Build history of the part. All positions in model axes, mm. Face numbers are marked on the shaded views. Round coordinates to 2 decimals unless told otherwise and drop trailing zeros. Loops run counter-clockwise (first coordinate to the right, second up) from the corner with the lowest first, then second, coordinate; pieces in that order, holes last. Notation, with made-up numbers: (-23.75, 35) - (18.25, 35) arc R12 ccw to (18.25, 53) - close; hole circle Ø6 at (-11.75, -11). An arc over 180 degrees is marked (long way). Use a Markdown table: item, result.
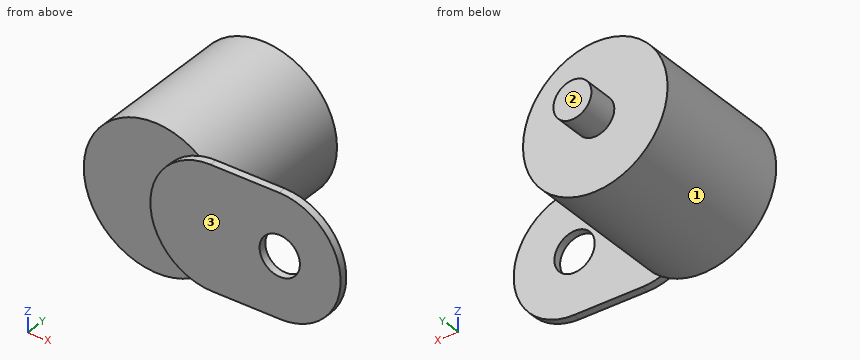
from build123d import *

# Parameters (mm, degrees)
SKETCH1_R           = 9.5
SKETCH1_R_2         = 2.5
BOSS_EXTRUDE1_DEPTH = 19
SKETCH2_R           = 2.5
BOSS_EXTRUDE2_DEPTH = 4
SKETCH3_R           = 2.65
BOSS_EXTRUDE3_DEPTH = 1


with BuildPart() as part:
    # Sketch1 → Boss-Extrude1 (new body)
    # profile 1 of 2: a face of its own
    with BuildSketch(Plane(origin=(0, 0, 0), x_dir=(1, 0, 0), z_dir=(0, 1, 0))):
        with Locations(Location((0, 0, 0), (0, 0, 270))):
            Circle(SKETCH1_R)
        Circle(SKETCH1_R_2, mode=Mode.SUBTRACT)
    # profile 2 of 2: a face of its own
    with BuildSketch(Plane(origin=(0, 0, 0), x_dir=(1, 0, 0), z_dir=(0, 1, 0))):
        Circle(SKETCH1_R_2)
    extrude(amount=BOSS_EXTRUDE1_DEPTH)

    # Sketch2 → Boss-Extrude2 (add)
    with BuildSketch(Plane(origin=(0, 19, 0), x_dir=(1, 0, 0), z_dir=(0, 1, 0))):
        with Locations(Location((0, 0, 0), (0, 0, 270))):
            Circle(SKETCH2_R)
    extrude(amount=BOSS_EXTRUDE2_DEPTH)

    # Sketch3 → Boss-Extrude3 (add)
    with BuildSketch(Plane.XZ):
        with BuildLine():
            Line((7.903037426, 7.99941237), (16.903037426, 8.108503279))
            ThreePointArc((16.903037426, 8.108503279), (24.99941237, 0.206053483), (17.096962574, -7.890321461))
            Line((17.096962574, -7.890321461), (8.096962574, -7.99941237))
            ThreePointArc((8.096962574, -7.99941237), (0.00058763, -0.096962574), (7.903037426, 7.99941237))
        make_face()
        with Locations(Location((17, 0.109090909, 0), (0, 0, 270))):
            Circle(SKETCH3_R, mode=Mode.SUBTRACT)
    extrude(amount=BOSS_EXTRUDE3_DEPTH)


solid = part.part
Q1. Probe line 1 (Y direction, x = -0.5, z = 4); line 2 (Y direction, x = 15, z = -5); line 3 (X direction, y = 15.75, z = -3). List the from-to ranges inside material, lowest first.
Results found:
| item | result |
|---|---|
| line 1 | y = 0 to 19 |
| line 2 | y = -1 to 0 |
| line 3 | x = -9.01 to 9.01 |
Q2. Cut at B-B, the plane x = -2. List the corners of the cut face in (y, z).
Results found:
| item | result |
|---|---|
| outline | (0, -9.29) - (19, -9.29) - (19, -1.5) - (23, -1.5) - (23, 1.5) - (19, 1.5) - (19, 9.29) - (0, 9.29) - close |
Q3. Cut at D-D, the plane y = 21. List the corners of the cut face in (x, z).
Results found:
| item | result |
|---|---|
| outline | circle Ø5 at (0, 0) |
Q4. Pull direction Y, two halves, no side cores. Call the marked faces 1, 2 and 3: pulls with the +Y half, pulls with the -Y half, needs draft (parallel to the pull), parting line crosses it, or undercut.
Results found:
| item | result |
|---|---|
| face 1 | needs draft |
| face 2 | pulls with the +Y half |
| face 3 | pulls with the -Y half |
Q5. Cut at A-A, the plane z = 0. List the corners of the cut face in (x, y), plus the area to 3 significant figures.
Results found:
| item | result |
|---|---|
| outline | (-9.5, 0) - (0, 0) - (0, -1) - (14.35, -1) - (14.35, 0) - (9.5, 0) - (9.5, 19) - (2.5, 19) - (2.5, 23) - (-2.5, 23) - (-2.5, 19) - (-9.5, 19) - close; (19.65, -1) - (25, -1) - (25, 0) - (19.65, 0) - close |
| area | 401 mm2 |
Q6. Drop flat-ended pins along their axis: pin 1 (5.5 mm diameter, centred on x = 0.5, z = 4, fed in from +Y); pin 2 (1.5 mm diameter, centred on x = 14, z = -5.5, fed in from +Y); pin 3 (5 mm diameter, centred on y = 6.5, z = -6, fed in from +X); pin 4 (2 mm diameter, centred on x = 1.5, z = -4.5, fed in from +Y). Give the stop position or say it passes through.
Results found:
| item | result |
|---|---|
| pin 1 | stops at y = 23 |
| pin 2 | stops at y = 0 |
| pin 3 | stops at x = 8.83 |
| pin 4 | stops at y = 19 |
Q7. Cut at C-C, the plane z = -7. List the corners of the cut face in (x, y).
Results found:
| item | result |
|---|---|
| outline | (-6.42, 0) - (4.13, 0) - (4.13, -1) - (20.67, -1) - (20.67, 0) - (6.42, 0) - (6.42, 19) - (-6.42, 19) - close |
